Input: dimensioned drawing with shaded views. Units: mm. Origin: part minimum x, y, z. Coordinates: 2 decimals unless noted, no trailing zeros. Loops run counter-clockwise (first coordinate to the right, second up) from the corner with the lowest first, then second, coordinate; pieces in that order, holes last.
(1) Line query: L1, parallel to X at y = 5, z = 8; L2, parallel to Y at x = 9, z = 6; L3, parallel to X at y = 11.75, z = 8.5. Output: solid intervals per line, ascending.
(2) Section C-C, the plane y = 9. Return loops of the section in (x, z), then the cut area to 3 significant figures.
(3) Section B-B, the plane x = 27. Return loops of the section in (y, z).
(4) Section D-D, the plane y = 11. Return loops of the section in (x, z).
(5) Section A-A, the plane z = 9. Return loops of the section in (x, y).
(6) Contact query for flat-ended pins moving along their axis: P1, Ø4, axis at y = 12, z = 13, coming from the -X side; P2, Ø2, axis at y = 13.5, z = 2, coming from the +X side (3 decimals); P3, Ø1.6, axis at x = 9, y = 11, coming from the -Z side. Output: stop coordinate, or through.
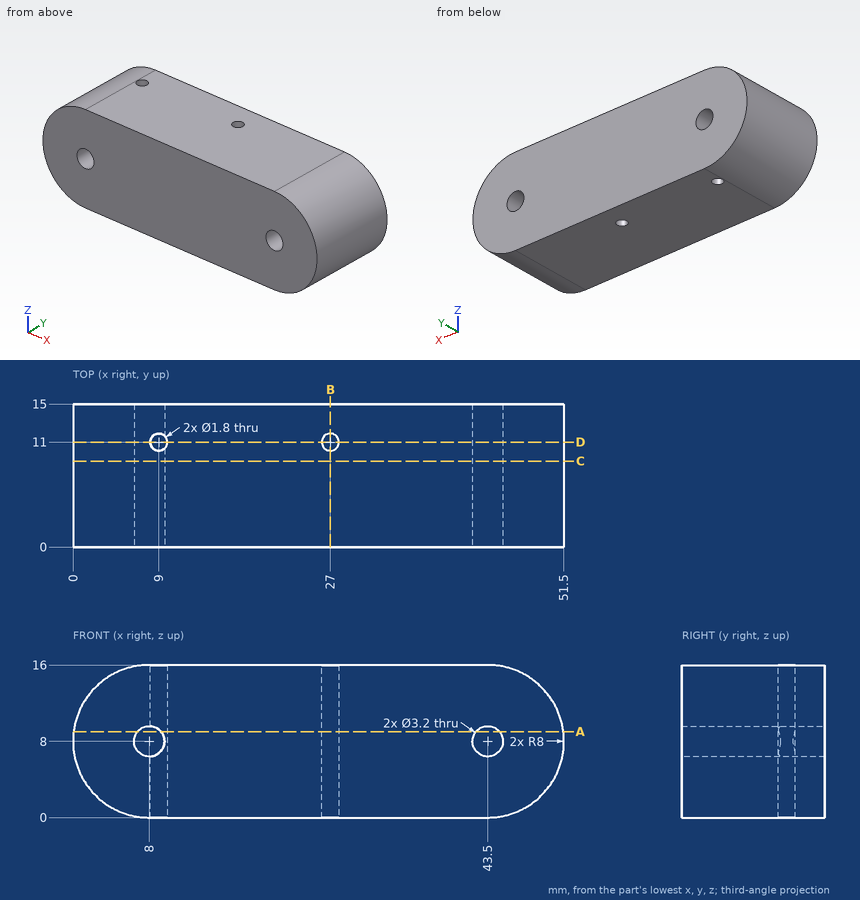
Report:
1. L1: x = 0 to 6.4, 9.6 to 41.9, 45.1 to 51.5
1. L2: y = 0 to 10.1, 11.9 to 15
1. L3: x = 0.02 to 6.48, 9.52 to 26.5, 27.5 to 41.98, 45.02 to 51.48
2. outline: (8, 0) - (43.5, 0) arc R8 ccw to (43.5, 16) - (8, 16) arc R8 ccw to start; hole circle Ø3.2 at (8, 8); hole circle Ø3.2 at (43.5, 8)
2. area: 753 mm2
3. outline: (0, 0) - (10.1, 0) - (10.1, 16) - (0, 16) - close; (11.9, 0) - (15, 0) - (15, 16) - (11.9, 16) - close
4. outline: (8, 0) - (8.1, 0) - (8.1, 6.4) arc R1.6 cw (long way) to (8.1, 9.6) - (8.1, 16) - (8, 16) arc R8 ccw to start; (9.9, 0) - (26.1, 0) - (26.1, 16) - (9.9, 16) - close; (27.9, 0) - (43.5, 0) arc R8 ccw to (43.5, 16) - (27.9, 16) - close; hole circle Ø3.2 at (43.5, 8)
5. outline: (0.06, 0) - (6.75, 0) - (6.75, 15) - (0.06, 15) - close; (9.25, 0) - (42.25, 0) - (42.25, 15) - (9.25, 15) - (9.25, 11.86) arc R0.9 cw to (9.25, 10.14) - close; (44.75, 0) - (51.44, 0) - (51.44, 15) - (44.75, 15) - close; hole circle Ø1.8 at (27, 11)
6. P1: stops at x = 0.58
6. P2: stops at x = 49.745
6. P3: passes through
